```python
from build123d import *

# Parameters (mm, degrees)
F0_W     = 88.9
F0_H     = 6.35
F1_DEPTH = 0.8128


with BuildPart() as f1:
    # F0 (on Front) → F1 (new body)
    with BuildSketch(Plane.XZ):
        with BuildLine():
            ThreePointArc((-241.3, 0), (-248.902375, -9.233938), (-260.35, -12.7))
            Line((-260.35, -12.7), (-260.35, -298.45))
            ThreePointArc((-260.35, -298.45), (-246.879616, -304.029616), (-241.3, -317.5))
            Line((-241.3, -317.5), (241.3, -317.5))
            ThreePointArc((241.3, -317.5), (246.879616, -304.029616), (260.35, -298.45))
            Line((260.35, -298.45), (260.35, -12.7))
            ThreePointArc((260.35, -12.7), (248.902375, -9.233938), (241.3, 0))
            Line((241.3, 0), (241.3, 76.2))
            ThreePointArc((241.3, 76.2), (247.223093, 91.60143), (260.35, 101.6))
            Line((260.35, 101.6), (260.35, 158.75))
            ThreePointArc((260.35, 158.75), (0, 419.1), (-260.35, 158.75))
            Line((-260.35, 158.75), (-260.35, 101.6))
            ThreePointArc((-260.35, 101.6), (-247.223093, 91.60143), (-241.3, 76.2))
            Line((-241.3, 76.2), (-241.3, 0))
        make_face()
        with Locations((-152.4, -47.625)):
            Rectangle(F0_W, F0_H, mode=Mode.SUBTRACT)
        with Locations((152.4, -47.625)):
            Rectangle(F0_W, F0_H, mode=Mode.SUBTRACT)
    extrude(amount=F1_DEPTH)


solid = f1.part
```
CAD build for the part. Positions are in the model's coordinates, mm. A direction names the side the tool comes from. Round coordinates to 2 decimals unless told otherwise and drop trailing zeros. Write each loop counter-clockwise with the first axis right and the second up, starting at its lowest first coordinate (ties: lowest second). Pieces come first, ordered by that corner, then holes. Notation, with made-up numbers: (-36, -1.5) -> (15, -1.5) arc R8 ccw to (15, 10.5) -> close; hole circle Ø8 at (-22.75, 57). An arc over 180 degrees is marked (long way). Answer in a Markdown table with one row per item. Add a question column.
Item 1: Saw through at C-C, the plane z = 40.5. Write the cut outline in (x, y), then the cut area to 3 significant figures.
Item 2: Saw through at A-A, the plane x = -129. Write the cut outline in (y, z), then the cut area to 3 significant figures.
Item 3: Which spindle directions (+Z, -Z, +X, -X, +Y, -Y) get a long thin tool onto all of the face, cutting with end or side? Do faces 1 (the face through (247.08, -0.4, 91.41)), 2 (the face through (-4, -0.813, 56)), 3 (the face through (-247.364, -0.401, 91.788)). Say none if no direction does.
Item 4: Saw through at B-B, the plane y = -0.4. Count the separate pieces of the cut face and the enclosed holes in it, then the cut area to 3 significant figures.
Item 5: Drill centre lines: line 1 (Z direction, x = 141, y = -0.65); line 2 (X direction, y = -0.6, z = 5.5); line 3 (Z direction, x = 179.5, y = -0.1). Where is each one in solid material? Low to high. Write a range as from..to.
Item 6: Saw through at D-D, the plane z = 344.5. Write the cut outline in (x, y), then the cut area to 3 significant figures.
Findings below:
| question | item | result |
|---|---|---|
| 1 | outline | (-241.3, -0.81) -> (241.3, -0.81) -> (241.3, 0) -> (-241.3, 0) -> close |
| 1 | area | 392 mm^2 |
| 2 | outline | (-0.81, -317.5) -> (0, -317.5) -> (0, -50.8) -> (-0.81, -50.8) -> close; (-0.81, -44.45) -> (0, -44.45) -> (0, 384.89) -> (-0.81, 384.89) -> close |
| 2 | area | 566 mm^2 |
| 3 | face 1 | +X, +Y, -Y |
| 3 | face 2 | +Z, -Z, +X, -X, -Y |
| 3 | face 3 | -X, +Y, -Y |
| 4 | separate pieces | 1 |
| 4 | enclosed holes | 2 |
| 4 | area | 349,000 mm^2 |
| 5 | line 1 | z = -317.5..-50.8, -44.45..377.61 |
| 5 | line 2 | x = -241.3..241.3 |
| 5 | line 3 | z = -317.5..-50.8, -44.45..347.33 |
| 6 | outline | (-182.43, -0.81) -> (182.43, -0.81) -> (182.43, 0) -> (-182.43, 0) -> close |
| 6 | area | 297 mm^2 |
